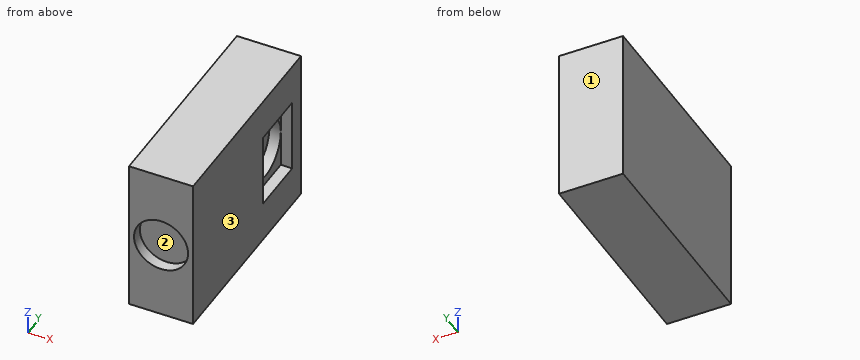
Autodesk Inventor part; units mm, degrees
ref_plane "YZ Plane" through (0, 0, 0) normal (1, 0, 0) x (0, 1, 0)
ref_plane "XZ Plane" through (0, 0, 0) normal (0, 1, 0) x (-1, 0, 0)
ref_plane "XY Plane" through (0, 0, 0) normal (0, 0, 1) x (1, 0, 0)
sketch "Skizze1" plane through (0, 0, 0) normal (1, 0, 0) x (0, 1, 0)
  line L0 (0, 0) -> (18.5, 0)
  line L1 (18.5, 0) -> (18.5, 13.6)
  line L2 (18.5, 13.6) -> (0, 13.6)
  line L3 (0, 13.6) -> (0, 0)
  dimension "d0" = 18.5
  dimension "d1" = 13.6
extrude "Extrusion1" add sketch "Skizze1" along normal blind 5.6
sketch "Skizze2" plane through (5.6, 0, 0) normal (1, 0, 0) x (0, 0, -1)
  line L0 (0, 18.5) -> (-13.6, 18.5)
  line L1 (-13.6, 18.5) -> (-13.6, 0)
  line L2 (-13.6, 0) -> (0, 0)
  line L3 (0, 0) -> (0, 18.5)
  line L4 (-10.05, 12) -> (-3.55, 12)
  line L5 (-3.55, 12) -> (-3.55, 17)
  line L6 (-3.55, 17) -> (-10.05, 17)
  line L7 (-10.05, 17) -> (-10.05, 12)
  line L8 (-10.05, 12) -> (-3.55, 17) construction
  line L9 (-3.55, 12) -> (-10.05, 17) construction
  point P0 (-6.8, 14.5)
  dimension "d4" = 6.5
  dimension "d5" = 5
  dimension "d6" = 1.5
extrude "Extrusion2" cut sketch "Skizze2" against normal blind 1 contours L7 L6 L5 L4
sketch "Skizze3" plane through (0, 0, 0) normal (0, -1, 0) x (1, 0, 0)
  line L0 (0, 13.6) -> (0, 0)
  line L1 (0, 0) -> (5.6, 0)
  line L2 (5.6, 13.6) -> (5.6, 0)
  line L3 (0, 13.6) -> (5.6, 13.6)
  circle A0 centre (2.8, 6.8) radius 2.3625
extrude "Extrusion3" cut sketch "Skizze3" against normal blind 1 contours A0
sketch "Skizze4" plane through (4.6, 0, 0) normal (1, 0, 0) x (0, 0, -1)
  line L0 (-3.55, 17) -> (-3.55, 12)
  line L1 (-10.05, 17) -> (-3.55, 17)
  line L2 (-10.05, 12) -> (-10.05, 17)
  line L3 (-3.55, 12) -> (-10.05, 12)
  circle A0 centre (-6.8, 14.5) radius 2.5
  point P0 (0, 0)
extrude "Extrusion4" cut sketch "Skizze4" against normal blind 1 contours A0
ref_plane "Arbeitsebene1" through (2.8, 0, 0) normal (-1, 0, 0) x (0, 0, 1)
properties part number "00_huawei_p30_Objectivelensassembly"
Check sheet for the modelled part. Datum: model origin and axes. Units: mm. Face numbers are marked on the shaded views. Coordinates: 2 decimals unless noted, no trailing zeros. Write each loop counter-clockwise with the first axis right and the second up, starting at its lowest first coordinate (ties: lowest second). Pieces come first, ordered by that corner, then holes. Notation, with made-up numbers: (-24.5, 22) - (20.5, 22) arc R19 cw to (20.5, 26) - close; hole circle Ø7 at (50.25, -15.5). An arc over 180 degrees is marked (long way). One line per question, with ' | ' between items.
Item 1: Mould release check, pull along X, two halves, no side actions. Record for the marked faces 1, 2 and 3: pulls with the +X half, pulls with the -X half, needs draft (parallel to the pull), parting line crosses it, or undercut.
Determined:
face 1: needs draft | face 2: undercut | face 3: pulls with the +X half
Item 2: Gauge pin test, flat ends, axial feed: P1, Ø3, axis at y = 14.5, z = 6.8, coming from the +X side; P2, Ø1.4, axis at x = 2.5, z = 5.5, coming from the -Y side. Record the tip position at first contact, or that the pin passes through.
Determined:
P1: stops at x = 3.6 | P2: stops at y = 1
Item 3: Sectioned sample at B-B on y = 12.5. Record the boundary of the cut face in (x, z), plus the area to 3 significant figures.
Determined:
outline: (0, 0) - (5.6, 0) - (5.6, 3.55) - (4.6, 3.55) - (4.6, 5.3) - (3.6, 5.3) - (3.6, 8.3) - (4.6, 8.3) - (4.6, 10.05) - (5.6, 10.05) - (5.6, 13.6) - (0, 13.6) - close | area: 66.7 mm2
Item 4: Sectioned sample at C-C on x = 2.8. Record the boundary of the cut face in (y, z), plus the area to 3 significant figures.
Determined:
outline: (0, 0) - (18.5, 0) - (18.5, 13.6) - (0, 13.6) - (0, 9.16) - (1, 9.16) - (1, 4.44) - (0, 4.44) - close | area: 247 mm2
Item 5: Sectioned sample at A-A on x = 4.95. Record the boundary of the cut face in (y, z).
Determined:
outline: (0, 0) - (18.5, 0) - (18.5, 13.6) - (0, 13.6) - (0, 7.78) - (1, 7.78) - (1, 5.82) - (0, 5.82) - close; hole (12, 3.55) - (17, 3.55) - (17, 10.05) - (12, 10.05) - close
Item 6: Thickness scan on line 1 (Y direction, x = 4.3, z = 6.8); line 2 (Z direction, x = 3.9, y = 14.5); line 3 (Y direction, x = 5.25, z = 5.75). Record the ranges inside material, lowest first. Write a range as [from, to].
Determined:
line 1: y = [1, 12], [17, 18.5] | line 2: z = [0, 4.3], [9.3, 13.6] | line 3: y = [0, 12], [17, 18.5]
Item 7: Sectioned sample at D-D on z = 5.25. Record the boundary of the cut face in (x, y).
Determined:
outline: (0, 0) - (1.02, 0) - (1.02, 1) - (4.58, 1) - (4.58, 0) - (5.6, 0) - (5.6, 12) - (4.6, 12) - (4.6, 12.54) - (3.6, 12.54) - (3.6, 16.46) - (4.6, 16.46) - (4.6, 17) - (5.6, 17) - (5.6, 18.5) - (0, 18.5) - close
